Geometry: final body of the model. Coordinates: model frame, mm. A direction names the side the tool comes from. Give positions to 0.01 mm unless a question says otherwise; leave off trailing zeros. Write each loop counter-clockwise with the first axis right and the second up, starting at its lowest first coordinate (ties: lowest second). Pieces come first, ordered by that corner, then holes. Notation, with made-up numbers: (-39.75, -32.75) -> (-16.75, -32.75) arc R23 cw to (-16.75, -4.75) -> close; hole circle Ø10 at (42.5, -10). An arc over 180 degrees is marked (long way). Use CSV: the item, a comma, the result in double quotes. Start each with the question number.
1) Section B-B (z = 11.5). Output: boundary loops of the cut face in (x, y), plus the area to 3 significant figures.
2) Draft query along Z for faces 6 (the face through (-6, 3.5, 11)), 7 (the face through (-2, -9, 11)), 8 (the face through (-2, 8, 11)), 9 (the face through (-4, 0, 21)). Return one class per face: pulls with the +Z half, pulls with the -Z half, needs draft (parallel to the pull), parting line crosses it, or undercut.
3) Material intervals for line 1 (Z direction, x = -1.45, y = 8.5) (3 decimals); line 2 (X direction, y = 13, z = 3); line 3 (Y direction, x = -14.75, z = 1.75), sorted ascending. Write a range as [from, to].
4) Section A-A (x = -4.5). Output: boundary loops of the cut face in (y, z) (3 decimals), plus the area to 3 significant figures.
5) Contact query for flat-ended pins moving along their axis: P1, Ø2.5, axis at y = -8.5, z = 10.5, coming from the +X side; P2, Ø1.9, axis at x = -6.5, z = 9.5, coming from the +Y side; P3, Ø4, axis at y = 1, z = 14.5, coming from the +X side; P4, Ø1.9, axis at x = -6.5, z = 12, coming from the -Y side. Output: stop coordinate, or through.
6) Set-up query: faces 1 (the face through (-2, -17.25, 10)), 2 (the face through (-5, 15, 11)), 3 (the face through (-11.31, -8.66, 2.25)), 4 (the face through (-5, 0, 13)), 5 (the face through (-14.37, 10.56, 10.65)). Return all of +Z, -Z, +X, -X, +Y, -Y with unobstructed straight access to the full face (end or side cutting, diameter ignored); none if empty.
7) Section C-C (z = 16). Output: boundary loops of the cut face in (x, y), plus the area to 3 significant figures.
```python
from build123d import *

# Parameters (mm, degrees)
SKETCH007_W     = 34.5
SKETCH007_H     = 21
SKETCH007_R     = 1.925
PAD001_DEPTH    = 5
SKETCH008_R     = 1.925
POCKET006_DEPTH = 2
PAD002_DEPTH    = 21
SKETCH010_R     = 1.925
POCKET007_DEPTH = 2
SKETCH011_R     = 1.925
POCKET008_DEPTH = 24.335471


with BuildPart() as cono:
    # Cone → Cone (revolve)
    with BuildSketch(Plane(origin=(-17.5, 0, 0), x_dir=(1, 0, 0), z_dir=(0, -1, 0))):
        Polygon((0, 0), (10.415, 0), (11.6, 21), (0, 21), align=None)
    revolve(axis=Axis((-17.5, 0, 0), (0, 0, 1)))


with BuildPart() as obj1:
    # Sketch007 → Pad001 (new body)
    with BuildSketch(Plane.YZ):
        with Locations((0, 10.5)):
            Rectangle(SKETCH007_W, SKETCH007_H)
        with Locations((0, 10.5)):
            Circle(SKETCH007_R, mode=Mode.SUBTRACT)
    extrude(amount=-PAD001_DEPTH)

    # Sketch008 → Pocket006 (cut)
    with BuildSketch(Plane.YZ):
        with Locations((-8.5, 10.5)):
            Circle(SKETCH008_R)
        with Locations((8.5, 10.5)):
            Circle(SKETCH008_R)
    extrude(amount=-POCKET006_DEPTH, mode=Mode.SUBTRACT)

    # Sketch009 → Pad002 (new body)
    with BuildSketch(Plane(origin=(0, 0, 21), x_dir=(0, -1, 0), z_dir=(0, 0, 1))):
        with BuildLine():
            ThreePointArc((15.728159, -24.334314), (-8.6e-05, 0), (-15.728089, -24.334471))
            Line((-7.75, -24.334314), (-15.728089, -24.334471))
            ThreePointArc((-3.5, -7.350505), (-10.185925, -14.701091), (-7.75, -24.334314))
            Line((-3.5, -4), (-3.5, -7.350505))
            Line((3.5, -4), (-3.5, -4))
            Line((3.5, -7.350505), (3.5, -4))
            ThreePointArc((7.75, -24.334314), (10.185925, -14.701091), (3.5, -7.350505))
            Line((7.75, -24.334314), (15.728159, -24.334314))
        make_face()
    extrude(amount=-PAD002_DEPTH)

    # Sketch010 → Pocket007 (cut)
    with BuildSketch(Plane.YZ):
        with Locations((-8.5, 10.5)):
            Circle(SKETCH010_R)
        with Locations((8.5, 10.5)):
            Circle(SKETCH010_R)
    extrude(amount=-POCKET007_DEPTH, mode=Mode.SUBTRACT)

    # Sketch011 → Pocket008 (cut, through all)
    with BuildSketch(Plane.YZ):
        with Locations((0, 10.5)):
            Circle(SKETCH011_R)
    extrude(amount=-POCKET008_DEPTH, mode=Mode.SUBTRACT)

    # Cut: cut Cono
    add(cono.part, mode=Mode.SUBTRACT)


solid = obj1.part
```
Answers follow:
1,outline,"(-24.33, -15.73) arc R17.25 ccw to (-5, -12.14) -> (-5, -17.25) -> (0, -17.25) -> (0, -10.14) -> (-2, -10.14) -> (-2, -6.86) -> (0, -6.86) -> (0, -1.64) -> (-5, -1.64) -> (-5, -3.5) -> (-7, -3.5) arc R11.06 cw to (-24.33, -8.7) -> close; (-24.33, 8.7) arc R11.06 cw to (-7, 3.5) -> (-5, 3.5) -> (-5, 1.64) -> (0, 1.64) -> (0, 6.86) -> (-2, 6.86) -> (-2, 10.14) -> (0, 10.14) -> (0, 17.25) -> (-5, 17.25) -> (-5, 12.14) arc R17.25 ccw to (-24.33, 15.73) -> close"
1,area,"419 mm^2"
2,face 6,"needs draft"
2,face 7,"undercut"
2,face 8,"undercut"
2,face 9,"pulls with the +Z half"
3,line 1,"z = [0, 8.575], [12.425, 21]"
3,line 2,"x = [-24.33, -5.91], [-5, 0]"
3,line 3,"y = [-17.07, -10.2], [10.2, 17.07]"
4,outline,"(-17.25, 0) -> (17.25, 0) -> (17.25, 21) -> (-17.25, 21) -> close; hole circle Ø3.85 at (0, 10.5)"
4,area,"713 mm^2"
5,P1,"stops at x = -2"
5,P2,"stops at y = 14.2"
5,P3,"stops at x = 0"
5,P4,"stops at y = -14.2"
6,face 1,"+Z, -Z, +X, -X, -Y"
6,face 2,"+Z, -Z, +Y"
6,face 3,"+Z, -Z"
6,face 4,"+Z, -Z, -X"
6,face 5,"+Z"
7,outline,"(-24.33, -15.73) arc R17.25 ccw to (-5, -12.14) -> (-5, -17.25) -> (0, -17.25) -> (0, 17.25) -> (-5, 17.25) -> (-5, 12.14) arc R17.25 ccw to (-24.33, 15.73) -> (-24.33, 9.02) arc R11.32 cw to (-6.74, 3.5) -> (-5, 3.5) -> (-5, -3.5) -> (-6.74, -3.5) arc R11.32 cw to (-24.33, -9.02) -> close"
7,area,"438 mm^2"
